from build123d import *

# Parameters (mm, degrees)
F5_DEPTH  = 38.1
F8_DEPTH  = 30.734
F9_W      = 7.62
F9_H      = 15.24
F9_W_2    = 10.16
F10_DEPTH = 25.4


# Not quite as in the source:
# - a feature of the source that left no trace in its solid (it failed there, or was rolled back) is left out


with BuildPart() as f5:
    # F3 (on face) → F5 (new body)
    with BuildSketch(Plane.XZ.offset(38.1)):
        with BuildLine():
            Line((0, 5.08), (0, 0))
            add(Edge.make_bspline(
                [(0, 0), (12.7, 0.707683037), (38.1, 2.1230491111), (63.5, 0.707683037), (76.2, 0)],
                knots=[0, 0, 0, 0, 0.5, 1, 1, 1, 1], degree=3))
            Line((76.2, 0), (76.2, 5.08))
            add(Edge.make_bspline(
                [(0, 5.08), (17.1016856021, 15.7050435078), (52.4364024312, 22.8591352455), (67.3437483547, 13.2911519776), (76.2, 5.08)],
                knots=[0, 0, 0, 0, 0.5766084835, 1, 1, 1, 1], degree=3))
        make_face()
    extrude(amount=-F5_DEPTH)

    # F7 (on offset) → F8 (cut)
    with BuildSketch(Plane.XY.offset(25.4)):
        with BuildLine():
            Line((0, -38.1), (38.1, -38.1))
            add(Edge.make_bspline(
                [(0, -36.195), (12.7, -37.1475), (25.4, -38.1), (38.1, -38.1)],
                knots=[0, 0, 0, 0, 0.5, 0.5, 0.5, 0.5], degree=3))
            Line((0, -36.195), (0, -38.1))
        make_face()
        with BuildLine():
            add(Edge.make_bspline(
                [(38.1, -38.1), (50.8, -38.1), (63.5, -37.1475), (76.2, -36.195)],
                knots=[0.5, 0.5, 0.5, 0.5, 1, 1, 1, 1], degree=3))
            Line((38.1, -38.1), (76.2, -38.1))
            Line((76.2, -38.1), (76.2, -36.195))
        make_face()
        with BuildLine():
            Line((76.2, 0), (38.1, 0))
            add(Edge.make_bspline(
                [(38.1, 0), (50.8, 0), (63.5, -0.9525), (76.2, -1.905)],
                knots=[0.5, 0.5, 0.5, 0.5, 1, 1, 1, 1], degree=3))
            Line((76.2, -1.905), (76.2, 0))
        make_face()
        with BuildLine():
            Line((38.1, 0), (0, 0))
            Line((0, 0), (0, -1.905))
            add(Edge.make_bspline(
                [(0, -1.905), (12.7, -0.9525), (25.4, 0), (38.1, 0)],
                knots=[0, 0, 0, 0, 0.5, 0.5, 0.5, 0.5], degree=3))
        make_face()
    extrude(amount=-F8_DEPTH, mode=Mode.SUBTRACT)

    # F9 (on offset) → F10 (cut)
    with BuildSketch(Plane.XY.offset(25.4)):
        with Locations((59.69, -11.43)):
            Rectangle(F9_W, F9_H)
        with Locations((59.69, -26.67)):
            Rectangle(F9_W, F9_H)
        with Locations((38.1, -26.67)):
            Rectangle(F9_W_2, F9_H)
        with Locations((38.1, -11.43)):
            Rectangle(F9_W_2, F9_H)
        with Locations((16.51, -26.67)):
            Rectangle(F9_W, F9_H)
        with Locations((16.51, -11.43)):
            Rectangle(F9_W, F9_H)
    extrude(amount=-F10_DEPTH, mode=Mode.SUBTRACT)


solid = f5.part
Input: part model. Units: mm. Frame: model coordinates. A direction names the side the tool comes from. Round coordinates to 2 decimals unless told otherwise and drop trailing zeros. Answer as a JSON object with one key per item and string values. Group by question number.
(1) Pin query (flat end, axial travel): P1, Ø5, axis at x = 41.5, y = -28.5, coming from the -Z side; P2, Ø6, axis at x = 17.5, z = 8, coming from the -Y side; P3, Ø6, axis at y = -14, z = 7, coming from the -X side; P4, Ø8.5, axis at x = 60, z = 7.5, coming from the +Y side. Return the tip coordinate at first contact, or that it passes through.
(2) Cut plane A-A (y = -33). Count the separate pieces of the cut face and the enclosed holes in it, then the cut area to 3 significant figures.
(3) Draft query along Y for faces 3 (the face through (38, -3.81, 10)), 4 (the face through (0, -19, 3)). Return one class per face: released by +Y, released by -Y, zero draft, split by the parting line, or undercut.
(4) Material intervals for probe 1 along X at (y, z) = (-18, 3.5); probe 2 along X at (y, z) = (-12, 12.25); probe 3 along X at (y, z) = (-22.5, 7.25), sorted ascending. Write a range as from..to.
(5) Reachability of faces 1 (the face through (43.18, -19, 10)), 2 (the face through (76.2, -19, 3)) from +Z, -Z, +X, -X, +Y, -Y: full face, straight path, thin tool, end or side. Return the list, or none.
Here are the results:
{
 "1": {"P1": "stops at z = 1.37", "P2": "stops at y = -37.58", "P3": "stops at x = 0", "P4": "stops at y = -0.52"},
 "2": {"separate pieces": "4", "enclosed holes": "0", "area": "638 mm^2"},
 "3": {"face 3": "undercut", "face 4": "zero draft"},
 "4": {"probe 1": "x = 0..12.7, 20.32..33.02, 43.18..55.88, 63.5..76.2", "probe 2": "x = 20.32..33.02, 43.18..55.88, 63.5..67.53", "probe 3": "x = 3.7..12.7, 20.32..33.02, 43.18..55.88, 63.5..73.81"},
 "5": {"face 1": "+Z, -Z", "face 2": "+Z, -Z, +X, +Y, -Y"}
}
